Geometry check sheet. Reference: the model listing, model coordinates, mm. A direction names the side the tool comes from. Coordinates: 2 decimals unless noted, no trailing zeros. Order: outer loops, then holes, each group sorted by start corner. A loop starts at its lowest first (then second) coordinate and runs counter-clockwise, first axis right, second up. Notation, with made-up numbers: (47, 58.5) -> (52, 58.5) arc R20 cw to (52, 96.5) -> close; hole circle Ø4 at (66.5, -29.75). An arc over 180 degrees is marked (long way). Answer as CSV lines item,"result". Start each with the question number.
from build123d import *

# Parameters (mm, degrees)
SKETCH1_W         = 19.05
SKETCH1_H         = 19.05
BODY_DEPTH        = 19.05
SLOT_DEPTH        = 12.7
BEVEL_LEFT_DEPTH  = 19.05
BEVEL_RIGHT_DEPTH = 19.05


with BuildPart() as part:
    # Sketch1 → Body (new body)
    with BuildSketch(Plane(origin=(0, 0, 0), x_dir=(1, 0, 0), z_dir=(0, 1, 0))):
        Rectangle(SKETCH1_W, SKETCH1_H)
    extrude(amount=BODY_DEPTH)

    # Sketch2 → Slot (cut)
    with BuildSketch(Plane(origin=(0, 19.05, 0), x_dir=(1, 0, 0), z_dir=(0, 1, 0))):
        Polygon((-2.3622, 9.525), (-2.3622, -2.3622), (9.525, -2.3622), (9.525, 0), (0, 0), (0, 9.525), align=None)
    extrude(amount=-SLOT_DEPTH, mode=Mode.SUBTRACT)

    # Sketch3 → Bevel Left (cut)
    with BuildSketch(Plane.XY.offset(9.525)):
        Polygon((-2.3622, 19.05), (-9.525, 19.05), (-9.525, 6.35), align=None)
    extrude(amount=-BEVEL_LEFT_DEPTH, mode=Mode.SUBTRACT)

    # Sketch4 → Bevel Right (cut)
    with BuildSketch(Plane(origin=(9.525, 0, 0), x_dir=(0, 0, -1), z_dir=(1, 0, 0))):
        Polygon((-2.3622, 19.05), (-9.525, 6.35), (-9.525, 19.05), align=None)
    extrude(amount=-BEVEL_RIGHT_DEPTH, mode=Mode.SUBTRACT)


solid = part.part
Q1. Sectioned sample at A-A, the plane y = 9. Record the cut outline in (x, z) (3 decimals), then the cut area to 3 significant figures.
Q2. Access from +Z, -Z, +X, -X, +Y, -Y to the whole of each face (thin tool, end or side, straight path). Record for faces 1 (the flat face through (0, 13, -5)), 2 (the flat face through (2, 7, -9.525)), 3 (the flat face through (5, 13, 0)).
Q3. Sectioned sample at D-D, the plane y = 16.5. Record the cut outline in (x, z) (3 decimals), then the cut area to 3 significant figures.
Q4. Release check for a two-part mould opening along X. For faces 4 (the flat face through (0, 0, 0)), 5 (the flat face through (0.9, 6.35, 0.3)), 6 (the flat face through (9.525, 7, -2)) record: released by +X, released by -X, zero draft, split by the parting line, or undercut.
Q5. Sectioned sample at B-B, the plane z = -6.25. Record the cut outline in (x, y) (3 decimals), then the cut area to 3 significant figures.
Q6. Thickness scan on L1, parallel to X at y = 17, z = -6.25 (3 decimals); L2, parallel to Y at x = 8.5, z = 0.5; L3, parallel to Z at x = 8.25, y = 10.5 (3 decimals). Record the ranges inside material, lowest first.
Q7. Sectioned sample at C-C, the plane x = 6.75. Record the cut outline in (y, z) (3 decimals), then the cut area to 3 significant figures.
Q8. Go/stop test with flat-tipped pins: pin 1 Ø2 at (x, z) = (6.5, -4.5) entering from -Y; pin 2 Ø10.5 at (x, y) = (6, 15.5) entering from +Z; pin 3 Ø3 at (y, z) = (15, -5.5) entering from -X; pin 4 Ø8 at (y, z) = (16.5, 6) entering from -X. Record where each tip stops, or that it passes through.
Geometry results:
1,outline,"(-8.03, -9.525) -> (-2.362, -9.525) -> (-2.362, 2.362) -> (9.525, 2.362) -> (9.525, 8.03) -> (-8.03, 8.03) -> close; (0, -9.525) -> (9.525, -9.525) -> (9.525, 0) -> (0, 0) -> close"
1,area,"258 mm^2"
2,face 1,"-Z, +Y"
2,face 2,"-Z, +X, -X, +Y, -Y"
2,face 3,"+X, +Y"
3,outline,"(-3.8, -9.525) -> (-2.362, -9.525) -> (-2.362, 2.362) -> (9.525, 2.362) -> (9.525, 3.8) -> (-3.8, 3.8) -> close; (0, -9.525) -> (9.525, -9.525) -> (9.525, 0) -> (0, 0) -> close"
3,area,"127 mm^2"
4,face 4,"zero draft"
4,face 5,"undercut"
4,face 6,"released by +X"
5,outline,"(-9.525, 0) -> (9.525, 0) -> (9.525, 19.05) -> (0, 19.05) -> (0, 6.35) -> (-2.362, 6.35) -> (-2.362, 19.05) -> (-9.525, 6.35) -> close"
5,area,"287 mm^2"
6,L1,"x = -3.518 to -2.362, 0 to 9.525"
6,L2,"y = 0 to 6.35"
6,L3,"z = -9.525 to 0, 2.362 to 7.184"
7,outline,"(0, -9.525) -> (19.05, -9.525) -> (19.05, 0) -> (6.35, 0) -> (6.35, 2.362) -> (19.05, 2.362) -> (6.35, 9.525) -> (0, 9.525) -> close"
7,area,"287 mm^2"
8,pin 1,"stops at y = 0"
8,pin 2,"stops at z = 7.33"
8,pin 3,"stops at x = -5.49"
8,pin 4,"stops at x = -6.06"
